```python
from build123d import *

# Parameters (mm, degrees)
F0_W     = 482.6
F0_H     = 88
F0_W_2   = 32.6
F0_H_2   = 24.3
F0_W_3   = 32
F0_W_4   = 37
F0_H_3   = 28.9
F0_W_5   = 17.2
F0_H_4   = 23
F0_W_6   = 17
F0_H_5   = 22.9
F0_R     = 10.25
F0_R_2   = 10.65
F0_W_7   = 27.5
F0_H_6   = 19.5
F1_DEPTH = 4
F2_D     = 5.5
F3_D     = 2.4


with BuildPart() as f1:
    # F0 (on Front) → F1 (new body)
    with BuildSketch(Plane.XZ):
        with Locations((-241.3, 44)):
            Rectangle(F0_W, F0_H)
        with BuildLine():
            ThreePointArc((-475.6, 2.15), (-479.35, 5.9), (-475.6, 9.65))
            Line((-475.6, 9.65), (-472.6, 9.65))
            ThreePointArc((-472.6, 9.65), (-468.85, 5.9), (-472.6, 2.15))
            Line((-472.6, 2.15), (-475.6, 2.15))
        make_face(mode=Mode.SUBTRACT)
        with Locations((-388.5, 26.05)):
            Rectangle(F0_W_2, F0_H_2, mode=Mode.SUBTRACT)
        with BuildLine():
            ThreePointArc((-10, 2.15), (-13.75, 5.9), (-10, 9.65))
            Line((-10, 9.65), (-7, 9.65))
            ThreePointArc((-7, 9.65), (-3.25, 5.9), (-7, 2.15))
            Line((-7, 2.15), (-10, 2.15))
        make_face(mode=Mode.SUBTRACT)
        with Locations((-141, 27.15)):
            Rectangle(F0_W_3, F0_H_2, mode=Mode.SUBTRACT)
        with Locations((-86, 27.15)):
            Rectangle(F0_W_3, F0_H_2, mode=Mode.SUBTRACT)
        with Locations((-388.5, 59.65)):
            Rectangle(F0_W_4, F0_H_3, mode=Mode.SUBTRACT)
        with Locations((-310, 44.05)):
            Rectangle(F0_W_5, F0_H_4, mode=Mode.SUBTRACT)
        with Locations((-278.5, 44)):
            Rectangle(F0_W_6, F0_H_5, mode=Mode.SUBTRACT)
        with Locations((-245, 44)):
            Circle(F0_R, mode=Mode.SUBTRACT)
        with BuildLine():
            ThreePointArc((-475.6, 78.35), (-479.35, 82.1), (-475.6, 85.85))
            Line((-475.6, 85.85), (-472.6, 85.85))
            ThreePointArc((-472.6, 85.85), (-468.85, 82.1), (-472.6, 78.35))
            Line((-472.6, 78.35), (-475.6, 78.35))
        make_face(mode=Mode.SUBTRACT)
        with Locations((-200, 44)):
            Circle(F0_R_2, mode=Mode.SUBTRACT)
        with Locations((-141, 60.85)):
            Rectangle(F0_W_7, F0_H_6, mode=Mode.SUBTRACT)
        with Locations((-86, 60.85)):
            Rectangle(F0_W_3, F0_H_2, mode=Mode.SUBTRACT)
        with BuildLine():
            ThreePointArc((-10, 78.35), (-13.75, 82.1), (-10, 85.85))
            Line((-10, 85.85), (-7, 85.85))
            ThreePointArc((-7, 85.85), (-3.25, 82.1), (-7, 78.35))
            Line((-7, 78.35), (-10, 78.35))
        make_face(mode=Mode.SUBTRACT)
    extrude(amount=F1_DEPTH)

    # F2 (through all)
    with Locations(Plane(origin=(0, 0, 0), x_dir=(1, 0, 0), z_dir=(0, 1, 0))):
        with Locations((-445.8, -80), (-445.8, -8), (-36.8, -80), (-36.8, -8)):
            Hole(F2_D / 2)

    # F3 (through all)
    with Locations(Plane(origin=(0, 0, 0), x_dir=(1, 0, 0), z_dir=(0, 1, 0))):
        with Locations((-121, -60.85), (-184.6, -44), (-215.4, -44), (-161, -60.85), (-278.5, -58.45), (-278.5, -29.55), (-365.75, -59.65), (-411.25, -59.65), (-409.55, -26.05), (-367.45, -26.05), (-106.15, -60.85), (-65.85, -60.85), (-65.85, -27.15), (-106.15, -27.15), (-310, -58.8), (-310, -29.8), (-161.15, -27.15), (-120.85, -27.15)):
            Hole(F3_D / 2)


solid = f1.part
```
Work out the finished part from the listing and answer in its coordinate system (mm). Give positions to 0.01 mm unless a question says otherwise; leave off trailing zeros. Loops run counter-clockwise (first coordinate to the right, second up) from the corner with the lowest first, then second, coordinate; pieces in that order, holes last. Notation, with made-up numbers: (15.5, 33) -> (53.5, 33) arc R32 ccw to (53.5, 69) -> close; hole circle Ø3 at (60, -24). An arc over 180 degrees is marked (long way). One line per question, with ' | ' between items. Start each with the question number.
1) Section B-B, the plane y = -3.3 is taken. State how many separate pieces and enclosed holes the cut face has, then the cut area to 3 significant figures.
2) Determine the mould class of faces 1 (the face through (-244.7, 0, 54.4)), 2 (the face through (-253.13, -1.97, 37.76)) for opening direction Z: +Z half, -Z half, draft (parallel to the pull), parting line (faces both ways), or undercut.
3) Section A-A, the plane x = -396.5 is taken. Determine the outline of the cut face in (y, z), then the cut area to 3 significant figures.
4) This flat-tipped pin is pushed along its axis until it touches: pin 1 (1.9 mm diameter, centred on x = -106.15, z = 60.85, fed in from -Y). Where does it stop, or does it pass through?
5) Straight lines are drawn through the part: L1, parallel to X at y = -1.3, z = 22; L2, parallel to Z at x = -128, y = -3.3; L3, parallel to Z at x = -310, y = -0.9. For each, find the intervals that lie inside material, in ascending order.
Resolved:
1) separate pieces: 1 | enclosed holes: 36 | area: 35,800 mm2
2) face 1: draft | face 2: undercut
3) outline: (-4, 0) -> (0, 0) -> (0, 13.9) -> (-4, 13.9) -> close; (-4, 38.2) -> (0, 38.2) -> (0, 45.2) -> (-4, 45.2) -> close; (-4, 74.1) -> (0, 74.1) -> (0, 88) -> (-4, 88) -> close | area: 139 mm2
4) pin 1: through
5) L1: -482.6 to -404.8, -372.2 to -157, -125 to -102, -70 to 0 | L2: 0 to 15, 39.3 to 51.1, 70.6 to 88 | L3: 0 to 28.6, 31 to 32.55, 55.55 to 57.6, 60 to 88
